Build history of the part. All positions in model axes, mm. A direction names the side the tool comes from. Give positions to 0.01 mm unless a question says otherwise; leave off trailing zeros. Order: outer loops, then holes, each group sorted by start corner. A loop starts at its lowest first (then second) coordinate and runs counter-clockwise, first axis right, second up. Notation, with made-up numbers: (48.5, -35.5) - (53.5, -35.5) arc R30 cw to (53.5, -4.5) - close; hole circle Ø6 at (42.5, -38). An arc over 180 degrees is marked (long way). Use a Markdown table: item, result.
Autodesk Inventor part; units mm, degrees
ref_plane "YZ Plane" through (0, 0, 0) normal (1, 0, 0) x (0, 1, 0)
ref_plane "XZ Plane" through (0, 0, 0) normal (0, 1, 0) x (-1, 0, 0)
ref_plane "XY Plane" through (0, 0, 0) normal (0, 0, 1) x (1, 0, 0)
ref_plane "Work Plane3" through (0, 0, 30) normal (0, 0, 1) x (1, 0, 0)
sketch "Sketch2" plane through (0, 0, 30) normal (0, 0, 1) x (1, 0, 0)
  circle A0 centre (0, 0) radius 12.15
  dimension "d12" = 24.3
extrude "Extrusion1" add sketch "Sketch2" along normal blind 46
chamfer "Chamfer2" distance 6 angle 45 1 edges at (-12.15, 0, 76)
sketch "Sketch3" plane through (0, 0, 30) normal (0, 0, -1) x (-1, 0, 0)
  circle A0 centre (0, 0) radius 12.15
  circle A1 centre (0, 0) radius 10
  dimension "d9" = 20
extrude "Extrusion2" add sketch "Sketch3" along normal blind 4 contours A1
properties part number "00_Microscope_Objective"
1) Pin check, flat tips, straight feed: P1, Ø10, axis at x = 8.5, z = 70, coming from the +Y side; P2, Ø5, axis at x = 6.5, y = -9.5, coming from the +Z side; P3, Ø1, axis at x = 8, z = 53, coming from the +Y side; P4, Ø10, axis at x = 0.5, z = 58.5, coming from the -Y side. Stop position of each tip, or through.
Computed:
| item | result |
|---|---|
| P1 | stops at y = 11.63 |
| P2 | stops at z = 73.14 |
| P3 | stops at y = 9.56 |
| P4 | stops at y = -12.15 |
2) Wall check: line 1 (X direction, y = -0.5, z = 57); line 2 (Z direction, x = -0.75, y = -8.25); line 3 (Y direction, x = 10.75, z = 40). Give the ranges that are in metal, low to high. Write a range as from..to.
Computed:
| item | result |
|---|---|
| line 1 | x = -12.14..12.14 |
| line 2 | z = 26..73.87 |
| line 3 | y = -5.66..5.66 |
3) Tool access for faces 1 (the flat face through (-10, -2, 30)), 2 (the flat face through (0, 0, 26)): list every direction of +Z, -Z, +X, -X, +Y, -Y with a clear straight run to the whole face (end or side of a thin tool).
Computed:
| item | result |
|---|---|
| face 1 | -Z |
| face 2 | -Z, +X, -X, +Y, -Y |
4) Slice it at A-A (y = 0). Write the cut outline in (x, z), and give its area (3 significant figures).
Computed:
| item | result |
|---|---|
| outline | (-12.15, 30) - (-10, 30) - (-10, 26) - (10, 26) - (10, 30) - (12.15, 30) - (12.15, 70) - (6.15, 76) - (-6.15, 76) - (-12.15, 70) - close |
| area | 1,160 mm² |
5) Slice it at C-C (z = 37). Write the cut outline in (x, y).
Computed:
| item | result |
|---|---|
| outline | circle Ø24.3 at (0, 0) |
